from build123d import *

# Parameters (mm, degrees)
CUT_EXTRUDE_2_DEPTH = 3
SKETCH_5_R          = 3.5
CUT_EXTRUDE_3_DEPTH = 107


with BuildPart() as part:
    # 草图2 → 旋转1 (revolve)
    with BuildSketch(Plane(origin=(0, 0, 0), x_dir=(1, 0, 0), z_dir=(0, 1, 0))):
        Polygon((0, 0), (0, 8), (15, 8), (15, 9), (92, 9), (92, 10), (98, 10), (98, 9), (106, 9), (106, 0), align=None)
    revolve(axis=Axis((0, 0, 0), (1, 0, 0)))

    # 草图4 → 切除-拉伸2 (cut)
    with BuildSketch(Plane.XY.offset(9)):
        with BuildLine():
            Line((62, 3), (87, 3))
            ThreePointArc((87, 3), (90, 0), (87, -3))
            Line((87, -3), (62, -3))
            ThreePointArc((62, -3), (59, 0), (62, 3))
        make_face()
    extrude(amount=-CUT_EXTRUDE_2_DEPTH, mode=Mode.SUBTRACT)

    # 草图5 → 切除-拉伸3 (cut, through all)
    with BuildSketch(Plane(origin=(106, 0, 0), x_dir=(0, 0, -1), z_dir=(1, 0, 0))):
        Circle(SKETCH_5_R)
    extrude(amount=-CUT_EXTRUDE_3_DEPTH, mode=Mode.SUBTRACT)


solid = part.part
Source: CAD feature listing. Evaluate the final solid. Frame: model axes, mm. A direction names the side the tool comes from. Give positions to 0.01 mm unless a question says otherwise; leave off trailing zeros. Order: outer loops, then holes, each group sorted by start corner. A loop starts at its lowest first (then second) coordinate and runs counter-clockwise, first axis right, second up. Notation, with made-up numbers: (36.5, 49.25) -> (65.5, 49.25) arc R21 cw to (65.5, 80.25) -> close; hole circle Ø7 at (11, 5.5). An arc over 180 degrees is marked (long way). Use a Markdown table: item, result.
1) Section query D-D, the plane z = -4.5. Return the cut outline in (x, y), then the cut area to 3 significant figures.
Answer list:
| item | result |
|---|---|
| outline | (0, -6.61) -> (15, -6.61) -> (15, -7.79) -> (92, -7.79) -> (92, -8.93) -> (98, -8.93) -> (98, -7.79) -> (106, -7.79) -> (106, 7.79) -> (98, 7.79) -> (98, 8.93) -> (92, 8.93) -> (92, 7.79) -> (15, 7.79) -> (15, 6.61) -> (0, 6.61) -> close |
| area | 1,630 mm² |
2) Reachability of faces 1 (the flat face through (0, -1.7, 3.4)), 2 (the flat face through (75, -3, 7)), 3 (the cylindrical face through (54.039, 2.703, -8.584)), 4 (the cylindrical face through (95.04, -9.76, 2.17)), 5 (the cylindrical face through (102.056, 8.923, 1.172)) from +Z, -Z, +X, -X, +Y, -Y: full face, straight path, thin tool, end or side. Return the list, or none.
Answer list:
| item | result |
|---|---|
| face 1 | +Z, -Z, -X, +Y, -Y |
| face 2 | +Z |
| face 3 | -X |
| face 4 | +X, -X |
| face 5 | +X |
3) Section query A-A, the plane y = 0. Return the cut outline in (x, z), then the cut area to 4 significant figures.
Answer list:
| item | result |
|---|---|
| outline | (0, -8) -> (15, -8) -> (15, -9) -> (92, -9) -> (92, -10) -> (98, -10) -> (98, -9) -> (106, -9) -> (106, -3.5) -> (0, -3.5) -> close; (0, 3.5) -> (106, 3.5) -> (106, 9) -> (98, 9) -> (98, 10) -> (92, 10) -> (92, 9) -> (90, 9) -> (90, 6) -> (59, 6) -> (59, 9) -> (15, 9) -> (15, 8) -> (0, 8) -> close |
| area | 1,055 mm² |
4) Mould query, pull axis X, two halves, no side actions, for faces 6 (the flat face through (92, 2, -9)), 7 (the flat face through (106, -4, 0)), 8 (the cylindrical face through (7.6, -7.81, 1.73)), 9 (the flat face through (75, 0, 6)). Classes: +X half, -X half, draft (parallel to the pull), parting line (faces both ways), or undercut.
Answer list:
| item | result |
|---|---|
| face 6 | -X half |
| face 7 | +X half |
| face 8 | draft |
| face 9 | undercut |
5) Ray query, line 1 along Y through (x, z) = (25.5, 0); line 2 along X through (y, z) = (-8.75, -3.25); line 3 along Y through (x, z) = (85, 1.5). Return the intervals inside material, ascending. Write a range as [from, to].
Answer list:
| item | result |
|---|---|
| line 1 | [-9, -3.5], [3.5, 9] |
| line 2 | [92, 98] |
| line 3 | [-8.87, -3.16], [3.16, 8.87] |
6) Contact query for flat-ended pins moving along their axis: P1, Ø0.7, axis at x = 71.5, z = 7, coming from the +Y side; P2, Ø12, axis at x = 27.5, y = 1.5, coming from the -Z side; P3, Ø12, axis at x = 26, y = 6, coming from the +Z side. Output: stop coordinate, or through.
Answer list:
| item | result |
|---|---|
| P1 | y = 6.06 |
| P2 | z = -9 |
| P3 | z = 9 |
7) Section query B-B, the plane z = 0. Return the cut outline in (x, y).
Answer list:
| item | result |
|---|---|
| outline | (0, -8) -> (15, -8) -> (15, -9) -> (92, -9) -> (92, -10) -> (98, -10) -> (98, -9) -> (106, -9) -> (106, -3.5) -> (0, -3.5) -> close; (0, 3.5) -> (106, 3.5) -> (106, 9) -> (98, 9) -> (98, 10) -> (92, 10) -> (92, 9) -> (15, 9) -> (15, 8) -> (0, 8) -> close |
8) Section query C-C, the plane x = 18. Return the cut outline in (y, z), then the cut area to 3 significant figures.
Answer list:
| item | result |
|---|---|
| outline | circle Ø18 at (0, 0); hole circle Ø7 at (0, 0) |
| area | 216 mm² |
